Design review of the part built by this model. Coordinates are the model's own, in mm. A direction names the side the tool comes from. Give positions to 0.01 mm unless a question says otherwise; leave off trailing zeros. Order: outer loops, then holes, each group sorted by start corner. A loop starts at its lowest first (then second) coordinate and runs counter-clockwise, first axis right, second up. Notation, with made-up numbers: (30, 6) -> (35, 6) arc R25 ccw to (35, 36) -> close; hole circle Ø4 at (-35, 61.5). An arc over 180 degrees is marked (long way). Return JSON: item names as keys, results as strings.
```python
from build123d import *

# Parameters (mm, degrees)
SKETCH_1_R          = 4
SKETCH_1_R_2        = 1.5
EXTRUDE_1_DEPTH     = 3
SKETCH_2_W          = 26
SKETCH_2_H          = 3
EXTRUDE_2_DEPTH     = 31
SKETCH_3_R          = 5
SKETCH_3_R_2        = 1.5
CUT_EXTRUDE_1_DEPTH = 40.115214431
FILLET_1_R          = 3


with BuildPart() as part:
    # 草图1 → 凸台-拉伸1 (new body)
    with BuildSketch(Plane.XY):
        with BuildLine():
            Line((-13, 0), (-13, -20))
            Line((-13, -20), (13, -20))
            Line((13, -20), (13, 0))
            ThreePointArc((13, 0), (0, 13), (-13, 0))
        make_face()
        Circle(SKETCH_1_R, mode=Mode.SUBTRACT)
        with Locations((-8.5, 0)):
            Circle(SKETCH_1_R_2, mode=Mode.SUBTRACT)
        with Locations(Location((8.5, 0, 0), (0, 0, 180))):
            Circle(SKETCH_1_R_2, mode=Mode.SUBTRACT)
    extrude(amount=EXTRUDE_1_DEPTH)

    # 草图2 → 凸台-拉伸2 (add)
    with BuildSketch(Plane.XY):
        with Locations((0, -18.5)):
            Rectangle(SKETCH_2_W, SKETCH_2_H)
    extrude(amount=-EXTRUDE_2_DEPTH)

    # 草图3 → 切除-拉伸1 (cut, through all)
    with BuildSketch(Plane(origin=(0, 0, 0), x_dir=(1, 0, 0), z_dir=(0, 1, 0))):
        with Locations(Location((0, 16, 0), (0, 0, 270))):
            Circle(SKETCH_3_R)
        with Locations(Location((-8, 23, 0), (0, 0, 270))):
            Circle(SKETCH_3_R_2)
        with Locations(Location((8, 23, 0), (0, 0, 270))):
            Circle(SKETCH_3_R_2)
        with Locations(Location((8, 9, 0), (0, 0, 270))):
            Circle(SKETCH_3_R_2)
        with Locations(Location((-8, 9, 0), (0, 0, 270))):
            Circle(SKETCH_3_R_2)
    extrude(amount=-CUT_EXTRUDE_1_DEPTH, mode=Mode.SUBTRACT)

    # 圆角1
    fillet_1_edges = [part.edges().sort_by_distance(p)[0] for p in [
        (0, -20, 3),
        (-13, -18.5, -31),
        (13, -18.5, -31),
        (0, -17, 0),
    ]]
    fillet(fillet_1_edges, radius=FILLET_1_R)


solid = part.part
```
Item 1: Wall thickness on L1, parallel to X at y = -17.95, z = -23; L2, parallel to X at y = -18.85, z = -16; L3, parallel to Y at x = -1, z = -4: over which ranges is each line inside the solid? List them lowest first. Write a range as [from, to].
Result set:
{"L1": "x = [-13, -9.5], [-6.5, 6.5], [9.5, 13]", "L2": "x = [-13, -5], [5, 13]", "L3": "y = [-20, -17]"}
Item 2: Add section D-D (y = -3.5). Give the boundary of the cut face in (x, z), plus the area to 3 significant figures.
Result set:
{"outline": "(-13, 0) -> (-1.94, 0) -> (-1.94, 3) -> (-13, 3) -> close; (1.94, 0) -> (13, 0) -> (13, 3) -> (1.94, 3) -> close", "area": "66.4 mm^2"}
Item 3: For pin 1 (3.5 mm diameter, centred on x = -8, z = -23, fed in from +Y); pin 2 (13 mm diameter, centred on x = 3, y = 6, fed in from -Z), all flat-tipped, find the tip position at first contact; note any pin that passes through.
Result set:
{"pin 1": "stops at y = -17", "pin 2": "stops at z = 0"}
Item 4: Machinability: for faces 4 (the face through (3, -3, 0)), 5 (the face through (0.18, -19.14, 2.1)), which of the approach directions +Z, -Z, +X, -X, +Y, -Y give a long, thin tool a straight path to every point of the face, cutting with its end or side? Answer none if there is none.
Result set:
{"face 4": "-Z, +X, -X, +Y", "face 5": "+Z, +X, -X, -Y"}
Item 5: Mouldability with a two-part tool opening along Z and no side actions: class faces 1 (the face through (13, -17.5, -7.8)), 2 (the face through (12.1, -18.48, -30.14)), 3 (the face through (-9.464, -18.479, -9.325)) as released by +Z, released by -Z, zero draft, split by the parting line, or undercut.
Result set:
{"face 1": "zero draft", "face 2": "released by -Z", "face 3": "undercut"}
Item 6: Add section C-C (z = -23). Give the boundary of the cut face in (x, y), plus the area to 3 significant figures.
Result set:
{"outline": "(-13, -20) -> (-9.5, -20) -> (-9.5, -17) -> (-13, -17) -> close; (-6.5, -20) -> (6.5, -20) -> (6.5, -17) -> (-6.5, -17) -> close; (9.5, -20) -> (13, -20) -> (13, -17) -> (9.5, -17) -> close", "area": "60.0 mm^2"}
Item 7: Add section B-B (x = 0). Give the boundary of the cut face in (y, z).
Result set:
{"outline": "(-20, -31) -> (-17, -31) -> (-17, -21) -> (-20, -21) -> close; (-20, -11) -> (-17, -11) -> (-17, -3) arc R3 cw to (-14, 0) -> (-4, 0) -> (-4, 3) -> (-17, 3) arc R3 ccw to (-20, 0) -> close; (4, 0) -> (13, 0) -> (13, 3) -> (4, 3) -> close"}
Item 8: Add section A-A (z = -19). Give the boundary of the cut face in (x, y), plus the area to 3 significant figures.
Result set:
{"outline": "(-13, -20) -> (-4, -20) -> (-4, -17) -> (-13, -17) -> close; (4, -20) -> (13, -20) -> (13, -17) -> (4, -17) -> close", "area": "54.0 mm^2"}
